```python
from build123d import *

# Parameters (mm, degrees)
F0_W     = 152.4
F0_H     = 406.4
F1_DEPTH = 0.254
F4_DEPTH = 0.255
F5_DEPTH = 0.255
F7_DEPTH = 0.255


with BuildPart() as f1:
    # F0 (on Top) → F1 (new body)
    with BuildSketch(Plane.XY):
        with Locations((0, 86.128879)):
            Rectangle(F0_W, F0_H)
    extrude(amount=F1_DEPTH)

    # F3 (on face) → F4 (cut, through all)
    with BuildSketch(Plane.XY.offset(0.254)):
        with BuildLine():
            Line((31.598285, 126.768879), (-31.901715, 126.768879))
            ThreePointArc((-31.901715, 126.768879), (-41.779997, 122.677161), (-45.871715, 112.798879))
            Line((-45.871715, 112.798879), (-45.871715, 49.298879))
            ThreePointArc((-45.871715, 49.298879), (-41.779997, 39.420598), (-31.901715, 35.328879))
            Line((-31.901715, 35.328879), (31.598285, 35.328879))
            ThreePointArc((31.598285, 35.328879), (41.476567, 39.420598), (45.568285, 49.298879))
            Line((45.568285, 49.298879), (45.568285, 112.798879))
            ThreePointArc((45.568285, 112.798879), (41.476567, 122.677161), (31.598285, 126.768879))
        make_face()
    extrude(amount=-F4_DEPTH, mode=Mode.SUBTRACT)

    # F2 (on face) → F5 (cut, through all)
    with BuildSketch(Plane.XY.offset(0.254)):
        with BuildLine():
            Line((30.973906, 263.928879), (-32.526094, 263.928879))
            ThreePointArc((-32.526094, 263.928879), (-42.404376, 259.837161), (-46.496094, 249.958879))
            Line((-46.496094, 249.958879), (-46.496094, 186.458879))
            ThreePointArc((-46.496094, 186.458879), (-42.404376, 176.580598), (-32.526094, 172.488879))
            Line((-32.526094, 172.488879), (30.973906, 172.488879))
            ThreePointArc((30.973906, 172.488879), (40.852188, 176.580598), (44.943906, 186.458879))
            Line((44.943906, 186.458879), (44.943906, 249.958879))
            ThreePointArc((44.943906, 249.958879), (40.852188, 259.837161), (30.973906, 263.928879))
        make_face()
    extrude(amount=-F5_DEPTH, mode=Mode.SUBTRACT)

    # F6 (on face) → F7 (cut, through all)
    with BuildSketch(Plane.XY.offset(0.254)):
        with BuildLine():
            Line((32.582681, -10.391121), (-30.917319, -10.391121))
            ThreePointArc((-30.917319, -10.391121), (-40.7956, -14.482839), (-44.887319, -24.361121))
            Line((-44.887319, -24.361121), (-44.887319, -87.861121))
            ThreePointArc((-44.887319, -87.861121), (-40.7956, -97.739402), (-30.917319, -101.831121))
            Line((-30.917319, -101.831121), (32.582681, -101.831121))
            ThreePointArc((32.582681, -101.831121), (42.460963, -97.739402), (46.552681, -87.861121))
            Line((46.552681, -87.861121), (46.552681, -24.361121))
            ThreePointArc((46.552681, -24.361121), (42.460963, -14.482839), (32.582681, -10.391121))
        make_face()
    extrude(amount=-F7_DEPTH, mode=Mode.SUBTRACT)


solid = f1.part
```
Source: CAD feature listing. Evaluate the final solid. Frame: model axes, mm. Round coordinates to 2 decimals unless told otherwise and drop trailing zeros. Loops run counter-clockwise (first coordinate to the right, second up) from the corner with the lowest first, then second, coordinate; pieces in that order, holes last.
(1) Section query C-C (y = -80). Output: boundary loops of the cut face in (x, z), and give its area (3 significant figures).
From the geometry:
outline: (-76.2, 0) - (-44.89, 0) - (-44.89, 0.25) - (-76.2, 0.25) - close; (46.55, 0) - (76.2, 0) - (76.2, 0.25) - (46.55, 0.25) - close
area: 15.5 mm2
(2) Material intervals for probe 1 along Y at (x, z) = (13.5, 0.1); probe 2 along X at (y, z) = (88, 0.2); probe 3 along X at (y, z) = (239.5, 0.2), sorted ascending.
From the geometry:
probe 1: y = -117.07 to -101.83, -10.39 to 35.33, 126.77 to 172.49, 263.93 to 289.33
probe 2: x = -76.2 to -45.87, 45.57 to 76.2
probe 3: x = -76.2 to -46.5, 44.94 to 76.2
(3) Section query B-B (z = 0.2). Output: boundary loops of the cut face in (x, y).
From the geometry:
outline: (-76.2, -117.07) - (76.2, -117.07) - (76.2, 289.33) - (-76.2, 289.33) - close; hole (-46.5, 186.46) arc R13.97 ccw to (-32.53, 172.49) - (30.97, 172.49) arc R13.97 ccw to (44.94, 186.46) - (44.94, 249.96) arc R13.97 ccw to (30.97, 263.93) - (-32.53, 263.93) arc R13.97 ccw to (-46.5, 249.96) - close; hole (-45.87, 49.3) arc R13.97 ccw to (-31.9, 35.33) - (31.6, 35.33) arc R13.97 ccw to (45.57, 49.3) - (45.57, 112.8) arc R13.97 ccw to (31.6, 126.77) - (-31.9, 126.77) arc R13.97 ccw to (-45.87, 112.8) - close; hole (-44.89, -87.86) arc R13.97 ccw to (-30.92, -101.83) - (32.58, -101.83) arc R13.97 ccw to (46.55, -87.86) - (46.55, -24.36) arc R13.97 ccw to (32.58, -10.39) - (-30.92, -10.39) arc R13.97 ccw to (-44.89, -24.36) - close
(4) Section query A-A (x = -23). Output: boundary loops of the cut face in (y, z).
From the geometry:
outline: (-117.07, 0) - (-101.83, 0) - (-101.83, 0.25) - (-117.07, 0.25) - close; (-10.39, 0) - (35.33, 0) - (35.33, 0.25) - (-10.39, 0.25) - close; (126.77, 0) - (172.49, 0) - (172.49, 0.25) - (126.77, 0.25) - close; (263.93, 0) - (289.33, 0) - (289.33, 0.25) - (263.93, 0.25) - close
